Autodesk Fusion 360 part; units mm, degrees
sketch "Sketch6" plane through (0, 0, 0) normal (1, 0, 0) x (0, 1, 0)
  circle A0 centre (0, 0) radius 13.825
  circle A1 centre (0, 0) radius 11
  line L0 (-14, 14) -> (14, 14)
  line L1 (14, 14) -> (14, -14)
  line L2 (14, -14) -> (-14, -14)
  line L3 (-14, -14) -> (-14, 14)
  line L4 (-14, 14) -> (14, -14) construction
  line L5 (14, 14) -> (-14, -14) construction
  dimension "d41" = 27.65
  dimension "d42" = 22
extrude "Extrude8" add sketch "Sketch6" along normal blind 20 contours A0
extrude "Extrude9" add sketch "Sketch6" against normal blind 30 contours A0 | L0 L1 L2 L3
fillet "Fillet1" radius 10 1 edges at (-30, 0, 14)
fillet "Fillet2" radius 10 1 edges at (-30, 0, -14)
sketch "Sketch7" plane through (0, 14, 0) normal (0, 1, 0) x (-1, 0, 0)
  arc A0 (20, -14) -> (30, -4) centre (20, -4) ccw
  line L0 (30, -4) -> (30, 4)
  arc A1 (30, 4) -> (20, 14) centre (20, 4) ccw
  line L1 (20, 14) -> (0, 14)
  line L2 (0, 14) -> (0, -14)
  line L3 (0, -14) -> (20, -14)
  line L4 (0, 14) -> (27.0711, -11.0711) construction
  circle A2 centre (24.6168, 0) radius 1.75
  line L5 (0, -14) -> (27.0711, 11.0711) construction
  line L6 (15.1168, 0) -> (24.6168, 0) construction
  dimension "d51" = 3.5
  dimension "d55" = 9.5
extrude "Extrude10" cut sketch "Sketch7" along normal mid plane 42 from surface at -14 contours A2
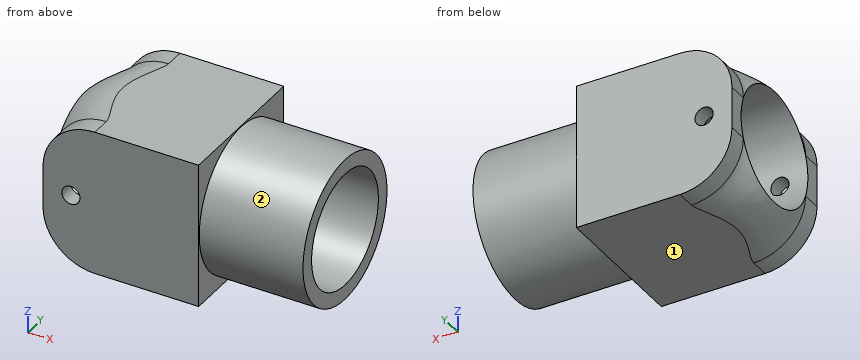
Work out the finished part from the listing and answer in its coordinate system (mm). Face numbers are marked on the shaded views. A direction names the side the tool comes from. Coordinates: 2 decimals unless noted, no trailing zeros. Write each loop counter-clockwise with the first axis right and the second up, starting at its lowest first coordinate (ties: lowest second). Pieces come first, ordered by that corner, then holes. Notation, with made-up numbers: M 14.25,-3.75 L 37.25,-3.75 A18 cw 37.25,3.25 Z; hole C 72,16.25 d6. An arc over 180 degrees is marked long. Use one line per item in the form item = value. Start each with the question number.
1. The part is cut by section C-C (x = 1). Give the vertices of the cut face in (y, z) (3 decimals), plus the area to 3 significant figures.
2. Straight lines are drawn through the part: probe 1 along Y at (x, z) = (-5, -0.25); probe 2 along Z at (x, y) = (1.5, 0) (3 decimals). For each, find the intervals that lie inside material, in ascending order. Write a range as from..to.
3. The part is cut by section B-B (x = -9.5). Give the vertices of the cut face in (y, z), plus the area to 3 significant figures.
4. The part is cut by section A-A (z = 0). Give the vertices of the cut face in (x, y) (3 decimals).
5. Each of these flat-tipped pins is pushed along its axis until it touches: P1, Ø3, axis at x = -24.62, z = 0, coming from the +Y side; P2, Ø8, axis at x = 10.5, y = -2.5, coming from the +Z side (3 decimals); P3, Ø3, axis at x = 14, z = 6.5, coming from the -Y side. Where does it stop, or does it pass through?
6. A tool of negligible diameter and unlimited length cuts with its end or side. For the marked faces 1 and 2, from which of +Z, -Z, +X, -X, +Y, -Y can it reach the whole face along a straight path? Write none if from no direction.
Evaluation:
q1.outline = C 0,0 d27.65; hole C 0,0 d22
q1.area = 220 mm^2
q2.probe_1 = -14..-11, 11..14
q2.probe_2 = -13.825..-11, 11..13.825
q3.outline = M -14,-14 L 14,-14 L 14,14 L -14,14 Z; hole C 0,0 d22
q3.area = 404 mm^2
q4.outline = M -30,-14 L -26.367,-14 L -26.367,-11 L -30,-11 Z; M -30,11 L -26.367,11 L -26.367,14 L -30,14 Z; M -22.867,-14 L 0,-14 L 0,-13.825 L 20,-13.825 L 20,-11 L -22.867,-11 Z; M -22.867,11 L 20,11 L 20,13.825 L 0,13.825 L 0,14 L -22.867,14 Z
q5.P1 = through
q5.P2 = 13.825
q5.P3 = -12.89
q6.face_1 = -Z, +X, -X, +Y, -Y
q6.face_2 = +X
